Work out the finished part from the listing and answer in its coordinate system (mm). Coordinates: 2 decimals unless noted, no trailing zeros. Loops run counter-clockwise (first coordinate to the right, second up) from the corner with the lowest first, then second, coordinate; pieces in that order, holes last. Notation, with made-up numbers: M 61.25,-7.75 L 106.25,-7.75 A19 ccw 106.25,19.25 Z; hole C 0.5,64 d11. An arc over 180 degrees is marked long. Write each question's results on one line, items separated by ' | '.
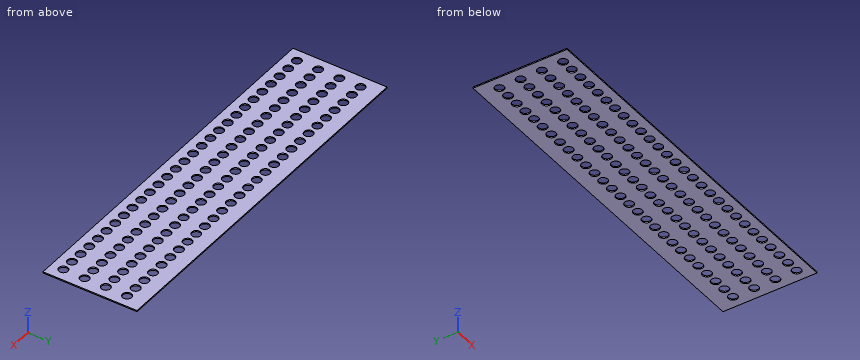
```python
from build123d import *

# Parameters (mm, degrees)
F1_W     = 303.5
F1_H     = 77.5
F2_DEPTH = 1
F0_R     = 3.75
F3_DEPTH = 25


with BuildPart() as f2:
    # F1 (on Top) → F2 (new body)
    with BuildSketch(Plane.XY):
        with Locations((141.75, 28.75)):
            Rectangle(F1_W, F1_H)
    extrude(amount=F2_DEPTH)

    # F0 (on Top) → F3 (cut)
    with BuildSketch(Plane.XY):
        with Locations((115.5, 17.5)):
            Circle(F0_R)
        with Locations((189, 17.5)):
            Circle(F0_R)
        with Locations((84, 0)):
            Circle(F0_R)
        with Locations((52.5, 35)):
            Circle(F0_R)
        with Locations((0, 35)):
            Circle(F0_R)
        with Locations((241.5, 17.5)):
            Circle(F0_R)
        with Locations((136.5, 0)):
            Circle(F0_R)
        with Locations((73.5, 35)):
            Circle(F0_R)
        with Locations((199.5, 0)):
            Circle(F0_R)
        with Locations((21, 35)):
            Circle(F0_R)
        with Locations((84, 17.5)):
            Circle(F0_R)
        with Locations((168, 0)):
            Circle(F0_R)
        with Locations((168, 35)):
            Circle(F0_R)
        with Locations((168, 17.5)):
            Circle(F0_R)
        with Locations((63, 0)):
            Circle(F0_R)
        with Locations((136.5, 35)):
            Circle(F0_R)
        with Locations((252, 17.5)):
            Circle(F0_R)
        with Locations((252, 35)):
            Circle(F0_R)
        with Locations((157.5, 17.5)):
            Circle(F0_R)
        with Locations((52.5, 0)):
            Circle(F0_R)
        with Locations((42, 17.5)):
            Circle(F0_R)
        with Locations((220.5, 17.5)):
            Circle(F0_R)
        with Locations((94.5, 0)):
            Circle(F0_R)
        with Locations((115.5, 35)):
            Circle(F0_R)
        with Locations((126, 17.5)):
            Circle(F0_R)
        with Locations((105, 35)):
            Circle(F0_R)
        with Locations((178.5, 17.5)):
            Circle(F0_R)
        with Locations((73.5, 0)):
            Circle(F0_R)
        with Locations((210, 35)):
            Circle(F0_R)
        with Locations((42, 35)):
            Circle(F0_R)
        with Locations((31.5, 17.5)):
            Circle(F0_R)
        with Locations((10.5, 17.5)):
            Circle(F0_R)
        with Locations((147, 17.5)):
            Circle(F0_R)
        with Locations((21, 0)):
            Circle(F0_R)
        with Locations((73.5, 17.5)):
            Circle(F0_R)
        with Locations((21, 17.5)):
            Circle(F0_R)
        with Locations((115.5, 0)):
            Circle(F0_R)
        with Locations((147, 35)):
            Circle(F0_R)
        with Locations((199.5, 17.5)):
            Circle(F0_R)
        with Locations((189, 0)):
            Circle(F0_R)
        with Locations((210, 17.5)):
            Circle(F0_R)
        with Locations((94.5, 35)):
            Circle(F0_R)
        with Locations((126, 35)):
            Circle(F0_R)
        with Locations((84, 35)):
            Circle(F0_R)
        with Locations((105, 0)):
            Circle(F0_R)
        with Locations((220.5, 35)):
            Circle(F0_R)
        with Locations((252, 0)):
            Circle(F0_R)
        with Locations((157.5, 35)):
            Circle(F0_R)
        with Locations((63, 17.5)):
            Circle(F0_R)
        with Locations((31.5, 0)):
            Circle(F0_R)
        with Locations((63, 35)):
            Circle(F0_R)
        with Locations((178.5, 35)):
            Circle(F0_R)
        with Locations((241.5, 0)):
            Circle(F0_R)
        with Locations((210, 0)):
            Circle(F0_R)
        with Locations((136.5, 17.5)):
            Circle(F0_R)
        with Locations((231, 17.5)):
            Circle(F0_R)
        with Locations((52.5, 17.5)):
            Circle(F0_R)
        with Locations((178.5, 0)):
            Circle(F0_R)
        with Locations((220.5, 0)):
            Circle(F0_R)
        with Locations((189, 35)):
            Circle(F0_R)
        with Locations((147, 0)):
            Circle(F0_R)
        with Locations((94.5, 17.5)):
            Circle(F0_R)
        with Locations((105, 17.5)):
            Circle(F0_R)
        with Locations((10.5, 35)):
            Circle(F0_R)
        with Locations((231, 0)):
            Circle(F0_R)
        with Locations((31.5, 35)):
            Circle(F0_R)
        with Locations((231, 35)):
            Circle(F0_R)
        with Locations((241.5, 35)):
            Circle(F0_R)
        with Locations((157.5, 0)):
            Circle(F0_R)
        with Locations((126, 0)):
            Circle(F0_R)
        with Locations((42, 0)):
            Circle(F0_R)
        with Locations((10.5, 0)):
            Circle(F0_R)
        with Locations((199.5, 35)):
            Circle(F0_R)
        with Locations((0, 17.5)):
            Circle(F0_R)
        Circle(F0_R)
        with Locations((262.5, 35)):
            Circle(F0_R)
        with Locations((273, 35)):
            Circle(F0_R)
        with Locations((283.5, 35)):
            Circle(F0_R)
        with Locations((283.5, 17.5)):
            Circle(F0_R)
        with Locations((273, 17.5)):
            Circle(F0_R)
        with Locations((262.5, 17.5)):
            Circle(F0_R)
        with Locations((262.5, 0)):
            Circle(F0_R)
        with Locations((273, 0)):
            Circle(F0_R)
        with Locations((283.5, 0)):
            Circle(F0_R)
        with Locations((63, 52.5)):
            Circle(F0_R)
        with Locations((94.5, 52.5)):
            Circle(F0_R)
        with Locations((10.5, 52.5)):
            Circle(F0_R)
        with Locations((168, 52.5)):
            Circle(F0_R)
        with Locations((73.5, 52.5)):
            Circle(F0_R)
        with Locations((31.5, 52.5)):
            Circle(F0_R)
        with Locations((126, 52.5)):
            Circle(F0_R)
        with Locations((21, 52.5)):
            Circle(F0_R)
        with Locations((105, 52.5)):
            Circle(F0_R)
        with Locations((115.5, 52.5)):
            Circle(F0_R)
        with Locations((157.5, 52.5)):
            Circle(F0_R)
        with Locations((42, 52.5)):
            Circle(F0_R)
        with Locations((52.5, 52.5)):
            Circle(F0_R)
        with Locations((147, 52.5)):
            Circle(F0_R)
        with Locations((136.5, 52.5)):
            Circle(F0_R)
        with Locations((84, 52.5)):
            Circle(F0_R)
        with Locations((0, 52.5)):
            Circle(F0_R)
        with Locations((283.5, 52.5)):
            Circle(F0_R)
        with Locations((210, 52.5)):
            Circle(F0_R)
        with Locations((231, 52.5)):
            Circle(F0_R)
        with Locations((220.5, 52.5)):
            Circle(F0_R)
        with Locations((273, 52.5)):
            Circle(F0_R)
        with Locations((262.5, 52.5)):
            Circle(F0_R)
        with Locations((178.5, 52.5)):
            Circle(F0_R)
        with Locations((189, 52.5)):
            Circle(F0_R)
        with Locations((199.5, 52.5)):
            Circle(F0_R)
        with Locations((241.5, 52.5)):
            Circle(F0_R)
        with Locations((252, 52.5)):
            Circle(F0_R)
    extrude(amount=F3_DEPTH, mode=Mode.SUBTRACT)


solid = f2.part
```
1) Find section A-A, the plane x = 10.5. Give the vertices of the cut face in (y, z).
Check result:
outline: M -10,0 L -3.75,0 L -3.75,1 L -10,1 Z; M 3.75,0 L 13.75,0 L 13.75,1 L 3.75,1 Z; M 21.25,0 L 31.25,0 L 31.25,1 L 21.25,1 Z; M 38.75,0 L 48.75,0 L 48.75,1 L 38.75,1 Z; M 56.25,0 L 67.5,0 L 67.5,1 L 56.25,1 Z
2) Find section B-B, the plane z = 0.35. Give the number of separate pieces and of enclosed holes in the cut face, and give its area (3 significant figures).
Check result:
separate pieces: 1 | enclosed holes: 112 | area: 18,600 mm^2
3) Given pin 1 Ø8.5 at (x, y) = (21, 17.5) entering from +Z, flat-ended and moving along its own axis, determine where the tip first touches the part or whether it passes through.
Check result:
pin 1: z = 1
4) Straight lines are drawn through the part: probe 1 along Y at (x, z) = (126, 0.5); probe 2 along Y at (x, z) = (8.5, 0.8). For each, find the intervals that lie inside material, in ascending order. Write a range as [from, to].
Check result:
probe 1: [-10, -3.75], [3.75, 13.75], [21.25, 31.25], [38.75, 48.75], [56.25, 67.5] | probe 2: [-10, -3.17], [3.17, 14.33], [20.67, 31.83], [38.17, 49.33], [55.67, 67.5]
